Work out the finished part from the listing and answer in its coordinate system (mm). A direction names the side the tool comes from. Coordinates: 2 decimals unless noted, no trailing zeros. Loops run counter-clockwise (first coordinate to the right, second up) from the corner with the lowest first, then second, coordinate; pieces in that order, holes last. Notation, with made-up numbers: (-20.5, 51.25) -> (20.5, 51.25) arc R17 cw to (20.5, 58.25) -> close; hole circle Ø2 at (78, -23.75). An arc over 180 degrees is marked (long way). Use a Markdown table: item, result. Add a question column.
```python
from build123d import *


with BuildPart() as part:
    # Esquisse1 → Révolution1 (revolve)
    with BuildSketch(Plane.XY):
        with BuildLine():
            Line((0, 0), (12, 0))
            Line((12, 0), (12, 2))
            Line((12, 2), (11.4, 2))
            Line((11.4, 2), (11.4, 3))
            Line((11.4, 3), (12, 3))
            Line((12, 3), (12, 11))
            Line((12, 11), (15.5, 11))
            Line((15.5, 11), (15.5, 15))
            Line((15.5, 15), (8, 17))
            ThreePointArc((8, 17), (4.472135955, 19.94427191), (0, 21))
            Line((0, 21), (0, 0))
        make_face()
    revolve(axis=Axis((0, 0, 0), (0, 1, 0)))


solid = part.part
```
Item 1: Section D-D (y = 13.25) is taken. Determine the outline of the cut face in (x, z).
Item 2: For a pull along Y with two mould halves and no side action, classify faces 4 (the face through (11, 2, 4)), 5 (the face through (-4.5, 11, 11.4)), 6 (the face through (-1.1, 16.9, -8.3)), 7 (the face through (-11.99, 1.01, -0.53)) as +Y half, -Y half, draft (parallel to the pull), parting line (faces both ways), or undercut.
Item 3: Section B-B (z = 0) is taken. Determine the outline of the cut face in (x, y).
Item 4: Find the intervals of material crossed by probe 1 along Z at (x, y) = (2, 14.25); probe 2 along Y at (x, z) = (-2.5, 8.5); probe 3 along X at (y, z) = (8.75, -9), in increasing order.
Item 5: Section C-C (y = 4.25) is taken. Determine the outline of the cut face in (x, z).
Item 6: Section A-A (x = 0) is taken. Determine the outline of the cut face in (y, z), then the cut area to 3 significant figures.
Item 7: For faces 1 (the face through (-11.99, 7.06, -0.53)), 2 (the face through (-9.047, 2.507, 6.937)), 3 (the face through (0, 0, 0)), determine the directions among +Z, -Z, +X, -X, +Y, -Y from which every point of the face is accessible in a straight line to the end or side of a thin tool.
Item 8: Given pin 1 (12 mm diameter, centred on y = 10, z = 10.5, fed in from +X); pin 2 (4 mm diameter, centred on x = 7.5, y = 7.5, fed in from +Z); pin 3 (10 mm diameter, centred on y = 13.5, z = -5.5, fed in from +X), each flat-ended and moving along its own axis, determine where each tip first touches the part or whether it passes through.
Output:
| question | item | result |
|---|---|---|
| 1 | outline | circle Ø31 at (0, 0) |
| 2 | face 4 | undercut |
| 2 | face 5 | -Y half |
| 2 | face 6 | +Y half |
| 2 | face 7 | draft |
| 3 | outline | (-15.5, 11) -> (-12, 11) -> (-12, 3) -> (-11.4, 3) -> (-11.4, 2) -> (-12, 2) -> (-12, 0) -> (12, 0) -> (12, 2) -> (11.4, 2) -> (11.4, 3) -> (12, 3) -> (12, 11) -> (15.5, 11) -> (15.5, 15) -> (8, 17) arc R10 ccw to (-8, 17) -> (-15.5, 15) -> close |
| 4 | probe 1 | z = -15.37 to 15.37 |
| 4 | probe 2 | y = 0 to 16.77 |
| 4 | probe 3 | x = -7.94 to 7.94 |
| 5 | outline | circle Ø24 at (0, 0) |
| 6 | outline | (0, -12) -> (2, -12) -> (2, -11.4) -> (3, -11.4) -> (3, -12) -> (11, -12) -> (11, -15.5) -> (15, -15.5) -> (17, -8) arc R10 ccw to (17, 8) -> (15, 15.5) -> (11, 15.5) -> (11, 12) -> (3, 12) -> (3, 11.4) -> (2, 11.4) -> (2, 12) -> (0, 12) -> close |
| 6 | area | 479 mm2 |
| 7 | face 1 | -Y |
| 7 | face 2 | none |
| 7 | face 3 | +Z, -Z, +X, -X, -Y |
| 8 | pin 1 | stops at x = 14.81 |
| 8 | pin 2 | stops at z = 10.67 |
| 8 | pin 3 | stops at x = 15.49 |
